Autodesk Inventor part; units mm, degrees
ref_plane "Work Plane1" through (-30, 0, -2) normal (1, 0, 0) x (0, 0, -1)
ref_plane "YZ Plane" through (0, 0, 0) normal (1, 0, 0) x (0, 1, 0)
ref_plane "XZ Plane" through (0, 0, 0) normal (0, 1, 0) x (-1, 0, 0)
sketch "Sketch1" plane through (0, 0, 0) normal (0, 1, 0) x (-1, 0, 0)
  line L0 (2, 0) -> (58, 0)
  line L1 (60, -2) -> (60, -87)
  line L2 (58, -89) -> (2, -89)
  line L3 (0, -87) -> (0, -2)
  arc A0 (60, -2) -> (58, 0) centre (58, -2) ccw
  arc A1 (2, 0) -> (0, -2) centre (2, -2) ccw
  arc A2 (58, -89) -> (60, -87) centre (58, -87) ccw
  arc A3 (0, -87) -> (2, -89) centre (2, -87) ccw
  point P0 (0, 0)
  point P1 (60, 0)
  point P2 (0, -89)
  dimension "d0" = 89
  dimension "d1" = 60
  dimension "d2" = 2
extrude "Extrusion1" add sketch "Sketch1" along normal blind 1
sketch "Sketch2" plane through (0, 1, 0) normal (0, 1, 0) x (1, 0, 0)
  line L0 (-60, 87) -> (-60, 2)
  line L1 (-58, 0) -> (-2, 0)
  line L2 (0, 2) -> (0, 87)
  line L3 (-2, 89) -> (-58, 89)
  line L4 (-2, 0) -> (-58, 0)
  line L5 (-60, 2) -> (-60, 87)
  line L6 (-58, 89) -> (-2, 89)
  line L7 (0, 87) -> (0, 2)
  arc A0 (-58, 89) -> (-60, 87) centre (-58, 87) ccw
  arc A1 (-60, 2) -> (-58, 0) centre (-58, 2) ccw
  arc A2 (-2, 0) -> (0, 2) centre (-2, 2) ccw
  arc A3 (0, 87) -> (-2, 89) centre (-2, 87) ccw
  line L8 (-55, 1.5) -> (-5, 1.5)
  line L9 (-1.5, 5) -> (-1.5, 84)
  line L10 (-5, 87.5) -> (-55, 87.5)
  line L11 (-58.5, 84) -> (-58.5, 5)
  arc A4 (-5, 1.5) -> (-1.5, 5) centre (-5, 5) ccw
  arc A5 (-58.5, 5) -> (-55, 1.5) centre (-55, 5) ccw
  arc A6 (-55, 87.5) -> (-58.5, 84) centre (-55, 84) ccw
  arc A7 (-1.5, 84) -> (-5, 87.5) centre (-5, 84) ccw
  point P0 (0, 0)
  point P1 (-60, 89)
  point P2 (-30, 89)
  point P3 (-2, 0)
  dimension "d5" = 2
  dimension "d6" = 1.5
  dimension "d7" = 1.5
  dimension "d8" = 1.5
  dimension "d9" = 1.5
  dimension "d10" = 3.5
extrude "Extrusion2" add sketch "Sketch2" along normal blind 9
sketch "Sketch4" plane through (0, 1, 0) normal (0, 1, 0) x (1, 0, 0)
  line L0 (-55, 1.5) -> (-5, 1.5)
  line L1 (-1.5, 5) -> (-1.5, 84)
  line L2 (-5, 87.5) -> (-55, 87.5)
  line L3 (-58.5, 84) -> (-58.5, 5)
  line L4 (-58.5, 5) -> (-58.5, 84)
  line L5 (-5, 1.5) -> (-55, 1.5)
  line L6 (-1.5, 84) -> (-1.5, 5)
  line L7 (-55, 87.5) -> (-5, 87.5)
  arc A0 (-55, 87.5) -> (-58.5, 84) centre (-55, 84) ccw
  arc A1 (-58.5, 5) -> (-55, 1.5) centre (-55, 5) ccw
  arc A2 (-5, 1.5) -> (-1.5, 5) centre (-5, 5) ccw
  arc A3 (-1.5, 84) -> (-5, 87.5) centre (-5, 84) ccw
  line L8 (-55, 2) -> (-5, 2)
  line L9 (-2, 5) -> (-2, 84)
  line L10 (-5, 87) -> (-55, 87)
  line L11 (-58, 84) -> (-58, 5)
  arc A4 (-58, 5) -> (-55, 2) centre (-55, 5) ccw
  arc A5 (-5, 2) -> (-2, 5) centre (-5, 5) ccw
  arc A6 (-2, 84) -> (-5, 87) centre (-5, 84) ccw
  arc A7 (-55, 87) -> (-58, 84) centre (-55, 84) ccw
  point P0 (0, 0)
  dimension "d13" = 3.5
  dimension "d14" = 0.5
  dimension "d15" = 0.5
  dimension "d16" = 0.5
  dimension "d17" = 0.5
  dimension "d18" = 3
  dimension "d19" = 3
extrude "Extrusion3" add sketch "Sketch4" along normal blind 2
sketch "Sketch5" plane through (0, 10, 0) normal (0, 1, 0) x (1, 0, 0)
  line L0 (-40, 0) -> (-20, 0)
  line L1 (-20, 0) -> (-20, 1.5)
  line L2 (-20.5, 2) -> (-39.5, 2)
  line L3 (-40, 1.5) -> (-40, 0)
  arc A0 (-39.5, 2) -> (-40, 1.5) centre (-39.5, 1.5) ccw
  arc A1 (-20, 1.5) -> (-20.5, 2) centre (-20.5, 1.5) ccw
  line L4 (-30, 0) -> (-30, 2) construction
  line L5 (-58, 0) -> (-2, 0) construction
  line L6 (-30, 0) -> (-30, 1.5) construction
  line L7 (-5, 1.5) -> (-55, 1.5) construction
  line L8 (-58, 0) -> (-2, 0) construction
  point P0 (0, 0)
  point P1 (-40, 2)
  dimension "d22" = 2
  dimension "d23" = 20
  dimension "d24" = 0.5
extrude "Extrusion4" cut sketch "Sketch5" against normal up to surface (10 mm away)
sketch "Sketch6" plane through (0, 0, -2) normal (1, 0, 0) x (0, 0, -1)
  line L0 (23.75, 10) -> (40.25, 10)
  line L1 (40.25, 10) -> (40.25, 6)
  line L2 (3, 3) -> (82, 3)
  line L3 (23.75, 10) -> (23.75, 6)
  line L4 (23.75, 6) -> (26.75, 4)
  line L5 (26.75, 4) -> (37.25, 4)
  line L6 (37.25, 4) -> (40.25, 6)
  line L7 (32, 10) -> (32, 4) construction
  line L8 (0, 10) -> (85, 10) construction
  line L9 (-2, 0) -> (-2, 10) construction
  dimension "d27" = 16.5
  dimension "d28" = 4
  dimension "d29" = 10.5
  dimension "d30" = 6
  dimension "d31" = 25.75
extrude "Extrusion5" cut sketch "Sketch6" against normal up to surface (1.5 mm away)
sketch "Sketch7" plane through (0, 0, -2) normal (1, 0, 0) x (0, 0, -1)
  line L0 (50, 10) -> (57, 10)
  line L1 (57, 10) -> (57, 7)
  line L2 (57, 7) -> (50, 7)
  line L3 (50, 7) -> (50, 10)
  line L4 (40.25, 10) -> (85, 10)
  arc A0 (50, 7) -> (57, 7) centre (53.5, 7) ccw
  line L5 (40.25, 10) -> (40.25, 6)
  point P0 (-2, 0)
  dimension "d34" = 7
  dimension "d35" = 3
  dimension "d36" = 9.75
extrude "Extrusion6" cut sketch "Sketch7" against normal up to surface (1.5 mm away)
sketch "Sketch8" plane through (0, 0, -2) normal (1, 0, 0) x (0, 0, -1)
  line L0 (6.5, 10) -> (14.7, 10)
  line L1 (14.7, 10) -> (14.7, 4.8)
  line L2 (14.7, 4.8) -> (6.5, 4.8)
  line L3 (6.5, 4.8) -> (6.5, 10)
  line L4 (6.5, 4.8) -> (7.3, 4)
  line L5 (7.3, 4) -> (13.9, 4)
  line L6 (13.9, 4) -> (14.7, 4.8)
  line L7 (0, 10) -> (23.75, 10)
  line L8 (23.75, 6) -> (23.75, 10)
  point P0 (-2, 0)
  point P1 (10.6, 4)
  dimension "d39" = 8.2
  dimension "d40" = 5.2
  dimension "d41" = 6.6
  dimension "d42" = 6
  dimension "d43" = 9.05
extrude "Extrusion7" cut sketch "Sketch8" against normal up to surface (1.5 mm away)
sketch "Sketch9" plane through (0, 0, -2) normal (1, 0, 0) x (0, 0, -1)
  line L0 (5.6855, 8.466) -> (15.5145, 8.466)
  line L1 (16.5145, 7.466) -> (16.5145, 4.078)
  line L2 (15.5145, 3.078) -> (5.6855, 3.078)
  line L3 (4.6855, 4.078) -> (4.6855, 7.466)
  arc A0 (5.6855, 8.466) -> (4.6855, 7.466) centre (5.6855, 7.466) ccw
  arc A1 (4.6855, 4.078) -> (5.6855, 3.078) centre (5.6855, 4.078) ccw
  arc A2 (15.5145, 3.078) -> (16.5145, 4.078) centre (15.5145, 4.078) ccw
  arc A3 (16.5145, 7.466) -> (15.5145, 8.466) centre (15.5145, 7.466) ccw
  line L4 (13.9, 4) -> (7.3, 4)
  line L5 (16.5145, 5.772) -> (14.7, 5.772) construction
  line L6 (14.7, 4.8) -> (14.7, 10) construction
  line L7 (4.6855, 5.772) -> (6.5, 5.772) construction
  line L8 (6.5, 10) -> (6.5, 4.8) construction
  point P0 (-2, 0)
  dimension "d46" = 5.388
  dimension "d47" = 11.829
  dimension "d48" = 1
  dimension "d49" = 0.922
extrude "Extrusion8" cut sketch "Sketch9" against normal blind 0.75
sketch "Sketch10" plane through (-2, 0, -89) normal (0, 0, -1) x (-1, 0, 0)
  line L0 (1.75, 10) -> (18.75, 10)
  line L1 (18.75, 10) -> (18.75, 4)
  line L2 (18.75, 4) -> (1.75, 4)
  line L3 (1.75, 4) -> (1.75, 10)
  line L4 (0, 10) -> (56, 10)
  line L5 (-2, 0) -> (-2, 10)
  dimension "d52" = 17
  dimension "d53" = 6
  dimension "d54" = 3.75
extrude "Extrusion9" cut sketch "Sketch10" against normal blind 2
sketch "Sketch11" plane through (-2, 0, -89) normal (0, 0, -1) x (-1, 0, 0)
  line L0 (21, 10) -> (37, 10)
  line L1 (37, 10) -> (37, 5.4)
  line L2 (37, 5.4) -> (36, 4.4)
  line L3 (36, 4.4) -> (22, 4.4)
  line L4 (22, 4.4) -> (21, 5.4)
  line L5 (21, 5.4) -> (21, 10)
  line L6 (29, 10) -> (29, 4.4) construction
  line L7 (18.75, 10) -> (56, 10) construction
  line L8 (18.75, 10) -> (18.75, 4) construction
  line L9 (55, 10) -> (55, 5.4)
  line L10 (39, 10) -> (55, 10)
  line L11 (39, 5.4) -> (39, 10)
  line L12 (40, 4.4) -> (39, 5.4)
  line L13 (54, 4.4) -> (40, 4.4)
  line L14 (55, 5.4) -> (54, 4.4)
  line L15 (37, 20) -> (37, 15.4)
  line L16 (21, 20) -> (37, 20)
  line L17 (21, 15.4) -> (21, 20)
  line L18 (22, 14.4) -> (21, 15.4)
  line L19 (36, 14.4) -> (22, 14.4)
  line L20 (37, 15.4) -> (36, 14.4)
  line L21 (55, 20) -> (55, 15.4)
  line L22 (39, 20) -> (55, 20)
  line L23 (39, 15.4) -> (39, 20)
  line L24 (40, 14.4) -> (39, 15.4)
  line L25 (54, 14.4) -> (40, 14.4)
  line L26 (55, 15.4) -> (54, 14.4)
  point P0 (-2, 0)
  point P1 (47, 10)
  point P2 (47, 4.4)
  point P3 (29, 20)
  point P4 (29, 14.4)
  point P5 (47, 20)
  point P6 (47, 14.4)
  dimension "d57" = 16
  dimension "d58" = 14
  dimension "d59" = 4.6
  dimension "d60" = 5.6
  dimension "d61" = 2.25
  dimension "d64" = 18
  dimension "d67" = 10
extrude "Extrusion10" cut sketch "Sketch11" against normal blind 2 contours L0 L1 L2 L3 L4 L5 | L9 L14 L13 L12 L11 L10
sketch "Sketch12" plane through (0, 0, 0) normal (0, -1, 0) x (1, 0, 0)
  arc A0 (0, -2) -> (-2, 0) centre (-2, -2) ccw
  line L0 (-2, 0) -> (-8, 0)
  line L1 (-8, 0) -> (-8, 6)
  line L2 (-8, 6) -> (-2, 6)
  line L3 (-2, 6) -> (-2, 0)
  circle A1 centre (-5, 6) radius 3
  circle A2 centre (-5, 6) radius 1.5
  arc A3 (-2, -89) -> (0, -87) centre (-2, -87) ccw
  line L4 (0, -87) -> (6, -87)
  line L5 (6, -87) -> (6, -81)
  line L6 (6, -81) -> (0, -81)
  line L7 (0, -81) -> (0, -87)
  circle A4 centre (6, -84) radius 3
  circle A5 centre (6, -84) radius 1.5
  point P0 (0, 0)
  dimension "d72" = 6
  dimension "d75" = 6
  dimension "d73" = 6
  dimension "d74" = 3
  dimension "d76" = 6
  dimension "d77" = 3
extrude "Extrusion11" add sketch "Sketch12" against normal blind 2 contours L0 L1 A1 L3 | A1 L2 A2 | L2 A2 A1 | L7 L6 A4 L4 | A4 L5 A5 | L5 A5 A4
ref_plane "Work Plane1" through (-30, 0, -2) normal (1, 0, 0) x (0, 0, -1)
mirror "Mirror1" about plane through (-30, 0, -2) normal (1, 0, 0) of "Extrusion11"
properties part number "raspi_enclosure"
Geometry: final body of the model. Coordinates: model frame, mm. A direction names the side the tool comes from. Coordinates: 2 decimals unless noted, no trailing zeros. Loops run counter-clockwise (first coordinate to the right, second up) from the corner with the lowest first, then second, coordinate; pieces in that order, holes last. Notation, with made-up numbers: (31.5, 38) -> (87.5, 38) arc R24 cw to (87.5, 68) -> close; hole circle Ø10 at (-17.5, -39). An arc over 180 degrees is marked (long way). Use a Markdown table: item, result. Add a question column.
(1) Access query for faces 4 (the flat face through (-58, 2, -45)), 5 (the flat face through (-55, 2, 4)), 6 (the flat face through (-2, 1, 3)). Directions: +Z, -Z, +X, -X, +Y, -Y. A direction counts if a zero-diameter tool reaches every point of the face in a straight line with its end or side. Return the directions, or none.
(2) Line query: line 1 along X through (y, z) = (0.7, -84); line 2 along X through (y, z) = (1.65, 6); line 3 along X through (y, z) = (1.65, -84). Output: solid intervals per line, ascending.
(3) Pin query (flat end, axial travel): pin 1 Ø5 at (y, z) = (5, -7.5) entering from -X; pin 2 Ø3 at (y, z) = (4.5, -47) entering from +X; pin 3 Ø4 at (x, y) = (-51, 3) entering from +Z; pin 4 Ø3.5 at (x, y) = (-31.5, 8) entering from +Z. Return the tip coordinate at first contact, or that it passes through.
(4) Mould query, pull axis X, two halves, no side actions, for faces 1 (the cylindrical face through (-59.43, 4.93, -88.4)), 2 (the flat face through (-1, 10, -74)), 3 (the cylindrical face through (5.805, 0.986, -82.513)). Classes: pulls with the +X half, pulls with the -X half, needs draft (parallel to the pull), parting line crosses it, or undercut.
(5) Section query D-D, the plane z = -44.5. Return loops of the section in (x, y).
(6) Section query A-A, the plane x = -28.5. Return loops of the section in (y, z), plus the area to 3 significant figures.
(7) Section query B-B, the plane z = -10.5. Return loops of the section in (x, y).
(8) Section query C-C, the plane x = -16. Return loops of the section in (y, z), plus the area to 3 significant figures.
Answer:
| question | item | result |
|---|---|---|
| 1 | face 4 | +Y |
| 1 | face 5 | +Z, +X, -X, +Y |
| 1 | face 6 | +Z, +X, +Y, -Y |
| 2 | line 1 | x = -69 to -67.5, -64.5 to 4.5, 7.5 to 9 |
| 2 | line 2 | x = -58 to -56.5, -53.5 to -52, -8 to -6.5, -3.5 to -2 |
| 2 | line 3 | x = -69 to -67.5, -64.5 to -58, -2 to 4.5, 7.5 to 9 |
| 3 | pin 1 | stops at x = -60 |
| 3 | pin 2 | stops at x = 0 |
| 3 | pin 3 | stops at z = 7.96 |
| 3 | pin 4 | passes through |
| 4 | face 1 | pulls with the -X half |
| 4 | face 2 | needs draft |
| 4 | face 3 | undercut |
| 5 | outline | (-60, 0) -> (0, 0) -> (0, 10) -> (-1.5, 10) -> (-1.5, 3) -> (-2, 3) -> (-2, 1) -> (-58, 1) -> (-58, 3) -> (-58.5, 3) -> (-58.5, 10) -> (-60, 10) -> close |
| 6 | outline | (0, -89) -> (4.4, -89) -> (4.4, -87.5) -> (3, -87.5) -> (3, -87) -> (1, -87) -> (1, -2) -> (0, -2) -> close |
| 6 | area | 93.1 mm^2 |
| 7 | outline | (-60, 0) -> (0, 0) -> (0, 3.08) -> (-0.75, 3.08) -> (-0.75, 4) -> (-1.5, 4) -> (-1.5, 3) -> (-2, 3) -> (-2, 1) -> (-58, 1) -> (-58, 3) -> (-58.5, 3) -> (-58.5, 10) -> (-60, 10) -> close |
| 8 | outline | (0, -89) -> (4, -89) -> (4, -87.5) -> (3, -87.5) -> (3, -87) -> (1, -87) -> (1, -2) -> (3, -2) -> (3, -1.5) -> (10, -1.5) -> (10, 0) -> (0, 0) -> close |
| 8 | area | 109 mm^2 |
